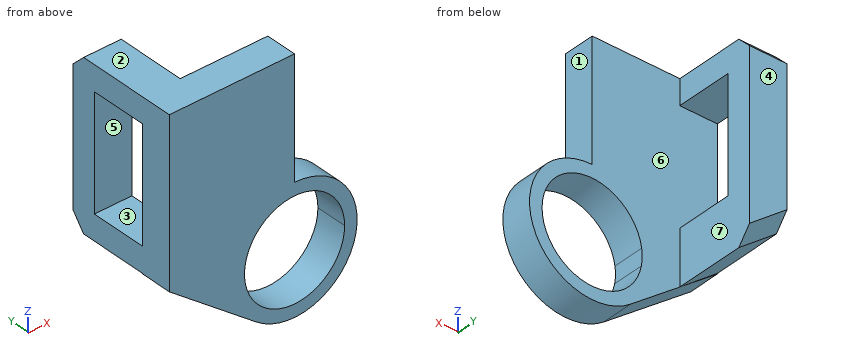
```python
from build123d import *

# Parameters (mm, degrees)
BOSS_EXTRUDE1_DEPTH = 6.35
SKETCH6_W           = 7.62
SKETCH6_H           = 5.08
BOSS_EXTRUDE3_DEPTH = 16.58
SKETCH8_W           = 7.62
SKETCH8_H           = 5.08
BOSS_EXTRUDE4_DEPTH = 23
CHAMFER1_SIZE       = 2.54


with BuildPart() as part:
    # Sketch1 → Boss-Extrude1 (new body)
    with BuildSketch(Plane(origin=(0, 0, 0), x_dir=(1, 0, 0), z_dir=(0, 1, 0))):
        with BuildLine():
            Line((0, -36.83), (0, -12.7))
            ThreePointArc((0, -12.7), (12.020636157, 4.098085697), (-7.757731828, 10.055227341))
            Line((-7.757731828, 10.055227341), (-25.4, -3.556))
            Line((-25.4, -3.556), (-25.4, -17.326729584))
            Line((-25.4, -17.326729584), (-25.4, -17.78))
            Line((-25.4, -17.78), (-25.4, -36.83))
            Line((-25.4, -36.83), (0, -36.83))
        make_face()
        with BuildLine():
            ThreePointArc((10.16, 0), (0.750509795, -10.13224235), (-10.049121072, -1.496918727))
            ThreePointArc((-10.049121072, -1.496918727), (-10.15820415, 0.191019487), (-9.985739115, 1.873663342))
            ThreePointArc((-9.985739115, 1.873663342), (0.940874749, 10.116340974), (10.16, 0))
        make_face(mode=Mode.SUBTRACT)
    extrude(amount=BOSS_EXTRUDE1_DEPTH)

    # Sketch6 → Boss-Extrude3 (add)
    with BuildSketch(Plane(origin=(0, 6.35, 0), x_dir=(1, 0, 0), z_dir=(0, 1, 0))):
        Polygon((-17.78, -3.67), (-17.78, 2.322923919), (-25.4, -3.67), align=None)
        with Locations((-21.59, -6.21)):
            Rectangle(SKETCH6_W, SKETCH6_H)
        with Locations((-21.59, -34.29)):
            Rectangle(SKETCH6_W, SKETCH6_H)
    extrude(amount=BOSS_EXTRUDE3_DEPTH)

    # Sketch8 → Boss-Extrude4 (add)
    with BuildSketch(Plane.XY.offset(8.75)):
        with Locations((-21.59, 20.39)):
            Rectangle(SKETCH8_W, SKETCH8_H)
    extrude(amount=BOSS_EXTRUDE4_DEPTH)

    # Chamfer1
    chamfer1_edges = [part.edges().sort_by_distance(p)[0] for p in [
        (-21.59, 22.93, 0.673538041),
        (-21.59, 22.93, 36.83),
    ]]
    chamfer(chamfer1_edges, length=CHAMFER1_SIZE)


solid = part.part
```
Work out the finished part from the listing and answer in its coordinate system (mm). Face numbers are marked on the shaded views. A direction names the side the tool comes from. Round coordinates to 2 decimals unless told otherwise and drop trailing zeros. Loops run counter-clockwise (first coordinate to the right, second up) from the corner with the lowest first, then second, coordinate; pieces in that order, holes last.
(1) Find the intervals of material crossed by L1, parallel to Y at x = -18, z = 13.5; L2, parallel to X at y = 6.5, z = 33.5; L3, parallel to X at y = 2, z = 24, in increasing order.
Computed values:
L1: y = 0 to 6.35, 17.85 to 22.93
L2: x = -25.4 to -17.78
L3: x = -25.4 to 0
(2) The part is cut by section A-A, the plane z = 20. Give the vertices of the cut face in (x, y).
Computed values:
outline: (-25.4, 0) - (0, 0) - (0, 6.35) - (-25.4, 6.35) - close; (-25.4, 17.85) - (-17.78, 17.85) - (-17.78, 22.93) - (-25.4, 22.93) - close
(3) The part is cut by section B-B, the plane y = 7. Give the vertices of the cut face in (x, z).
Computed values:
outline: (-25.4, 3.67) - (-17.78, -2.32) - (-17.78, 8.75) - (-25.4, 8.75) - close; (-25.4, 31.75) - (-17.78, 31.75) - (-17.78, 36.83) - (-25.4, 36.83) - close
(4) Each of these flat-tipped pins is pushed along its axis until it touches: P1, Ø7, axis at y = 2, z = 27.5, coming from the +X side; P2, Ø10, axis at x = 3, y = 12, coming from the -Z side; P3, Ø2, axis at x = -19, y = 20, coming from the -Z side; P4, Ø11.5, axis at x = 1, z = 6, coming from the +Y side. Where does it stop, or does it pass through?
Computed values:
P1: stops at x = 0
P2: passes through
P3: stops at z = -2.15
P4: stops at y = 6.35
(5) The part is cut by section C-C, the plane y = 1.5. Give the vertices of the cut face in (x, z), and give its area (3 significant figures).
Computed values:
outline: (-25.4, 3.56) - (-7.76, -10.06) arc R12.7 ccw (long way) to (0, 12.7) - (0, 36.83) - (-25.4, 36.83) - close; hole circle Ø20.32 at (0, 0)
area: 1,010 mm2
(6) The part is cut by section D-D, the plane x = -20.5. Give the vertices of the cut face in (y, z).
Computed values:
outline: (0, -0.22) - (6.35, -0.22) - (6.35, -0.18) - (20.39, -0.18) - (22.93, 3.05) - (22.93, 34.29) - (20.39, 36.83) - (0, 36.83) - close; hole (6.35, 8.75) - (17.85, 8.75) - (17.85, 31.75) - (6.35, 31.75) - close
(7) The mould has two halves that part along Y. Classify the marked faces 4, 5, 6 and 7: pulls with the +Y half, pulls with the -Y half, needs draft (parallel to the pull), parting line crosses it, or undercut.
Computed values:
face 4: pulls with the +Y half
face 5: undercut
face 6: undercut
face 7: needs draft
(8) For the marked faces 1, 2 and 3, determine the directions among +Z, -Z, +X, -X, +Y, -Y from which every point of the face is accessible in a straight line to the end or side of a thin tool.
Computed values:
face 1: +Z, +X, +Y, -Y
face 2: +Z, +X, -X, +Y, -Y
face 3: +X, -X
